Verification items for the finished model (mm, model axes). A direction names the side the tool comes from. Give positions to 0.01 mm unless a question says otherwise; leave off trailing zeros. Loops run counter-clockwise (first coordinate to the right, second up) from the corner with the lowest first, then second, coordinate; pieces in that order, holes last. Notation, with made-up numbers: (68.25, 81) -> (74.25, 81) arc R23 cw to (74.25, 102) -> close; hole circle Ø2 at (19.25, 33). An arc over 180 degrees is marked (long way). Answer in a Markdown table with one row per item. Add a question column.
Q1. Set-up check for faces 4 (the face through (41, 38, 44.5)), 5 (the face through (40.952, 72.794, 60.072)), 6 (the face through (-49.5, 38, 45)), 7 (the face through (38, 38, 73)), 8 (the face through (64.5, 38, 9)): record each of +Z, -Z, +X, -X, +Y, -Y from which the full face is reachable in a straight line by a thin tool's end or side.
Q2. Section check D-D on y = 22. Enter the section's corners in (x, z), and give its area (3 significant figures).
Q3. Gauge pin test, flat ends, axial feed: P1, Ø4.5, axis at x = 54.5, y = 49.5, coming from the +Z side; P2, Ø8, axis at y = 14, z = 64.5, coming from the -X side; P3, Ø6, axis at x = 42, y = 40.5, coming from the +Z side. Record the tip position at first contact, or that the pin passes through.
Q4. Section check B-B on y = 39. Enter the section's corners in (x, z), and give its area (3 significant figures).
Q5. Material ranges on probe 1 along X at (y, z) = (69, 32.5); probe 2 along Z at (x, y) = (46, 63); probe 3 along X at (y, z) = (65, 71.5), recorded low to high.
Q6. Release check for a two-part mould opening along Y. For faces 1 (the face through (49.5, 38, 31)), 2 (the face through (-15, 78, 15)), 3 (the face through (41.29, 35.01, 60.07)) record: pulls with the +Y half, pulls with the -Y half, needs draft (parallel to the pull), parting line crosses it, or undercut.
Q7. Section check C-C on x = 0. Enter the section's corners in (y, z), and give its area (3 significant figures).
Q8. Section check A-A on z = 38. Enter the section's corners in (x, y).
```python
from build123d import *

# Parameters (mm, degrees)
BOSS_EXTRUDE1_DEPTH          = 78
F_9_0_9_DIAMETER_HOLE1_D     = 9
F_9_0_9_DIAMETER_HOLE1_DEPTH = 25.5
M8_TAPPED_HOLE1_D            = 6.8
M8_TAPPED_HOLE1_DEPTH        = 19.75
M8_TAPPED_HOLE1_TIP          = 2.042926105


with BuildPart() as part:
    # Sketch1 → Boss-Extrude1 (new body)
    with BuildSketch(Plane(origin=(0, 0, 0), x_dir=(1, 0, 0), z_dir=(0, 1, 0))):
        with BuildLine():
            Line((-64.5, 0), (-64.5, -17))
            Line((-64.5, -17), (-49.5, -17))
            Line((-49.5, -17), (-49.5, -73))
            Line((-49.5, -73), (-37.242448899, -73))
            ThreePointArc((-37.242448899, -73), (0, -92), (37.242448899, -73))
            Line((37.242448899, -73), (49.5, -73))
            Line((49.5, -73), (49.5, -47.5))
            Line((49.5, -47.5), (32.465366161, -47.5))
            ThreePointArc((32.465366161, -47.5), (-32.5, -46), (32.465366161, -44.5))
            Line((32.465366161, -44.5), (49.5, -44.5))
            Line((49.5, -44.5), (49.5, -17))
            Line((49.5, -17), (64.5, -17))
            Line((64.5, -17), (64.5, 0))
            Line((64.5, 0), (0, 0))
            Line((0, 0), (-64.5, 0))
        make_face()
    extrude(amount=BOSS_EXTRUDE1_DEPTH)

    # Ø9.0 (9) Diameter Hole1
    with Locations(Plane.XY.offset(73)):
        with Locations((43.37122445, 69), (43.37122445, 39), (43.37122445, 9)):
            Hole(F_9_0_9_DIAMETER_HOLE1_D / 2, depth=F_9_0_9_DIAMETER_HOLE1_DEPTH)

    # M8 Tapped Hole1
    with Locations(Plane.XY.offset(44.5)):
        with Locations((43.37122445, 69), (43.37122445, 9)):
            Hole(M8_TAPPED_HOLE1_D / 2, depth=M8_TAPPED_HOLE1_DEPTH)
            with Locations((0, 0, -(M8_TAPPED_HOLE1_DEPTH + M8_TAPPED_HOLE1_TIP / 2))):  # 118° drill point
                Cone(0, M8_TAPPED_HOLE1_D / 2, M8_TAPPED_HOLE1_TIP, mode=Mode.SUBTRACT)


solid = part.part
```
Taken from the geometry:
| question | item | result |
|---|---|---|
| 1 | face 4 | +X, +Y, -Y |
| 1 | face 5 | +Z |
| 1 | face 6 | +Z, -X, +Y, -Y |
| 1 | face 7 | +Z, +X, +Y, -Y |
| 1 | face 8 | +Z, -Z, +X, +Y, -Y |
| 2 | outline | (-64.5, 0) -> (64.5, 0) -> (64.5, 17) -> (49.5, 17) -> (49.5, 44.5) -> (32.47, 44.5) arc R32.5 cw (long way) to (32.47, 47.5) -> (49.5, 47.5) -> (49.5, 73) -> (37.24, 73) arc R46 ccw to (-37.24, 73) -> (-49.5, 73) -> (-49.5, 17) -> (-64.5, 17) -> close |
| 2 | area | 5,360 mm² |
| 3 | P1 | stops at z = 17 |
| 3 | P2 | stops at x = -49.5 |
| 3 | P3 | stops at z = 73 |
| 4 | outline | (-64.5, 0) -> (64.5, 0) -> (64.5, 17) -> (49.5, 17) -> (49.5, 44.5) -> (32.47, 44.5) arc R32.5 cw (long way) to (32.47, 47.5) -> (38.87, 47.5) -> (38.87, 73) -> (37.24, 73) arc R46 ccw to (-37.24, 73) -> (-49.5, 73) -> (-49.5, 17) -> (-64.5, 17) -> close; (47.87, 47.5) -> (49.5, 47.5) -> (49.5, 73) -> (47.87, 73) -> close |
| 4 | area | 5,130 mm² |
| 5 | probe 1 | x = -49.5 to -29.56, 29.56 to 39.97, 46.77 to 49.5 |
| 5 | probe 2 | z = 0 to 44.5, 47.5 to 73 |
| 5 | probe 3 | x = -49.5 to -20.15, 20.15 to 41.31, 45.43 to 49.5 |
| 6 | face 1 | needs draft |
| 6 | face 2 | pulls with the +Y half |
| 6 | face 3 | undercut |
| 7 | outline | (0, 0) -> (78, 0) -> (78, 13.5) -> (0, 13.5) -> close; (0, 78.5) -> (78, 78.5) -> (78, 92) -> (0, 92) -> close |
| 7 | area | 2,110 mm² |
| 8 | outline | (-49.5, 0) -> (-31.5, 0) -> (-31.5, 78) -> (-49.5, 78) -> close; (31.5, 0) -> (49.5, 0) -> (49.5, 78) -> (31.5, 78) -> close; hole circle Ø6.8 at (43.37, 9); hole circle Ø6.8 at (43.37, 69) |
